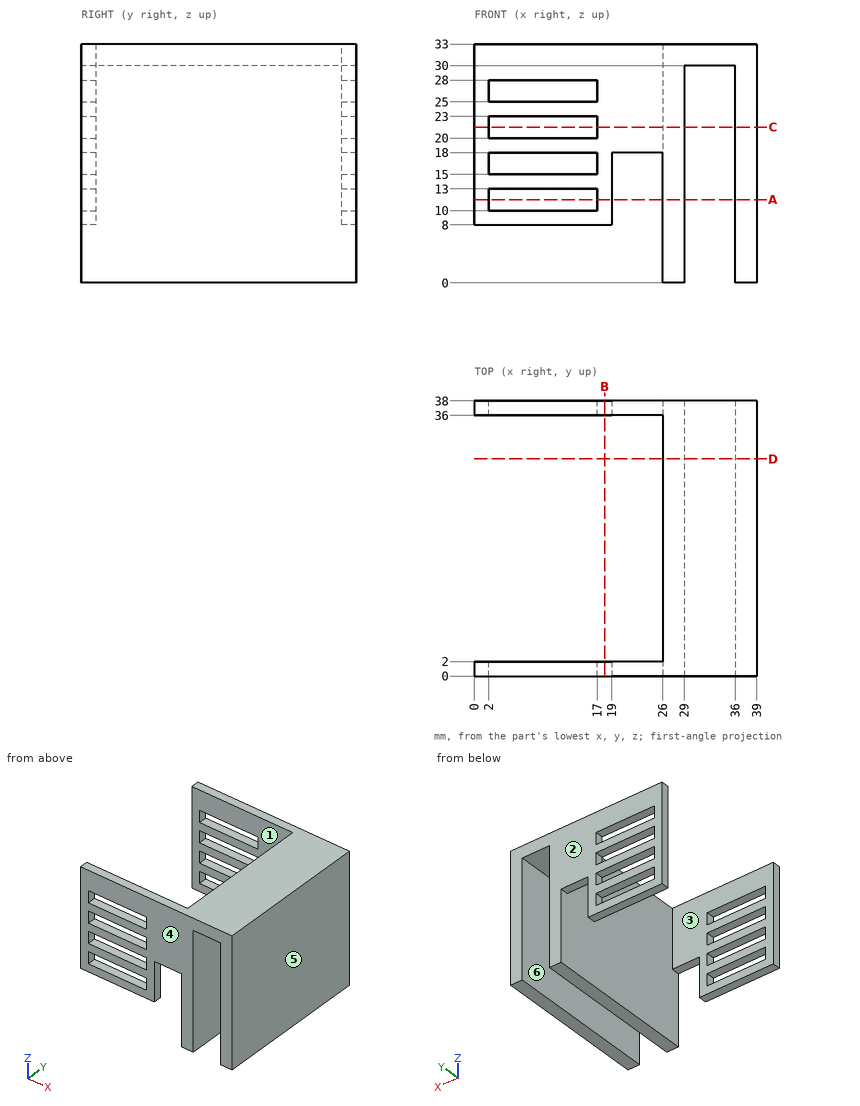
Part print with two shaded views. Sizes in mm from the minimum x, y, z corner. A direction names the side the tool comes from. Coordinates: 2 decimals unless noted, no trailing zeros. Order: outer loops, then holes, each group sorted by start corner. A loop starts at its lowest first (then second) coordinate and runs counter-clockwise, first axis right, second up. Notation, with made-up numbers: (29, 10.5) - (86, 10.5) arc R7 ccw to (86, 20.5) - close; hole circle Ø9 at (87, 29). An arc over 180 degrees is marked (long way). Write item = value, one per line. Start each with the question number.
1) Flat gauge pins, fed straight in: pin 1 Ø2 at (x, y) = (13, 37.5) entering from -Z; pin 2 Ø15 at (y, z) = (19, 8.5) entering from -X; pin 3 Ø2 at (x, y) = (34, 22) entering from -Z. Where does each tip first touch, or does it go through?
2) Saw through at C-C on z = 21.5. Write the cut outline in (x, y).
3) Saw through at A-A on z = 11.5. Write the cut outline in (x, y), then the cut area to 3 significant figures.
4) Saw through at B-B on x = 18. Write the cut outline in (y, z), then the cut area to 3 significant figures.
5) 3-axis set-ups, long thin cutter, end or side, ignore diameter. For the marked faces 5 and 6: which of +Z, -Z, +X, -X, +Y, -Y reach the whole face in a straight line?
6) Two-plate mould, pull along Y, no slides. Class the marked faces 1, 2, 3 and 4: pulls with the +Y half, pulls with the -Y half, needs draft (parallel to the pull), parting line crosses it, or undercut.
7) Wall check: line 1 along X through (y, z) = (3.5, 8.5); line 2 along Y through (x, z) = (17.5, 12.5); line 3 along X through (y, z) = (21.5, 31). Give the ranges that are in metal, low to high. Write a range as from..to.
8) Saw through at D-D on y = 30. Write the cut outline in (x, z), then the cut area to 3 significant figures.
From the geometry:
q1.pin_1 = 8
q1.pin_2 = 26
q1.pin_3 = 30
q2.outline = (0, 0) - (2, 0) - (2, 2) - (0, 2) - close; (0, 36) - (2, 36) - (2, 38) - (0, 38) - close; (17, 0) - (29, 0) - (29, 38) - (17, 38) - (17, 36) - (26, 36) - (26, 2) - (17, 2) - close; (36, 0) - (39, 0) - (39, 38) - (36, 38) - close
q3.outline = (0, 0) - (2, 0) - (2, 2) - (0, 2) - close; (0, 36) - (2, 36) - (2, 38) - (0, 38) - close; (17, 0) - (19, 0) - (19, 2) - (17, 2) - close; (17, 36) - (19, 36) - (19, 38) - (17, 38) - close; (26, 0) - (29, 0) - (29, 38) - (26, 38) - close; (36, 0) - (39, 0) - (39, 38) - (36, 38) - close
q3.area = 244 mm^2
q4.outline = (0, 8) - (2, 8) - (2, 33) - (0, 33) - close; (36, 8) - (38, 8) - (38, 33) - (36, 33) - close
q4.area = 100 mm^2
q5.face_5 = +Z, -Z, +X, +Y, -Y
q5.face_6 = -Z, +Y, -Y
q6.face_1 = undercut
q6.face_2 = pulls with the +Y half
q6.face_3 = undercut
q6.face_4 = pulls with the -Y half
q7.line_1 = 26..29, 36..39
q7.line_2 = 0..2, 36..38
q7.line_3 = 26..39
q8.outline = (26, 0) - (29, 0) - (29, 30) - (36, 30) - (36, 0) - (39, 0) - (39, 33) - (26, 33) - close
q8.area = 219 mm^2
